```python
from build123d import *

# Parameters (mm, degrees)
SKETCH2_R                       = 80
SKETCH2_R_2                     = 31
BOSS_EXTRUDE1_DEPTH             = 5
F_4_0MM_DOWEL_HOLE1_D           = 4
F_4_0MM_DOWEL_HOLE1_CSINK_D     = 4.05
F_4_0MM_DOWEL_HOLE1_CSINK_ANGLE = 90
F_3_0MM_DOWEL_HOLE1_D           = 3
F_3_0MM_DOWEL_HOLE1_CSINK_D     = 3.05
F_3_0MM_DOWEL_HOLE1_CSINK_ANGLE = 90
SKETCH13_R                      = 5
CUT_EXTRUDE1_DEPTH              = 3


with BuildPart() as part:
    # Sketch2 → Boss-Extrude1 (new body)
    with BuildSketch(Plane.XY):
        Circle(SKETCH2_R)
        Circle(SKETCH2_R_2, mode=Mode.SUBTRACT)
    extrude(amount=BOSS_EXTRUDE1_DEPTH)

    # Ø4.0mm Dowel Hole1 (through all)
    with Locations(Plane.XY.offset(5)):
        with Locations((0, 70), (-49.497474683, 49.497474683), (-70, 0), (-49.497474683, -49.497474683), (0, -70), (49.497474683, -49.497474683), (70, 0), (49.497474683, 49.497474683)):
            CounterSinkHole(F_4_0MM_DOWEL_HOLE1_D / 2, F_4_0MM_DOWEL_HOLE1_CSINK_D / 2, counter_sink_angle=F_4_0MM_DOWEL_HOLE1_CSINK_ANGLE)

    # Ø3.0mm Dowel Hole1 (through all)
    with Locations(Plane.XY.offset(5)):
        with Locations((0, 37), (-26.162950904, 26.162950904), (-37, 0), (-26.162950904, -26.162950904), (0, -37), (26.162950904, -26.162950904), (37, 0), (26.162950904, 26.162950904)):
            CounterSinkHole(F_3_0MM_DOWEL_HOLE1_D / 2, F_3_0MM_DOWEL_HOLE1_CSINK_D / 2, counter_sink_angle=F_3_0MM_DOWEL_HOLE1_CSINK_ANGLE)

    # Sketch13 → Cut-Extrude1 (cut)
    with BuildSketch(Plane.XY):
        with Locations((0, 37)):
            Circle(SKETCH13_R)
        with Locations((26.162950904, 26.162950904)):
            Circle(SKETCH13_R)
        with Locations((37, 0)):
            Circle(SKETCH13_R)
        with Locations((26.162950904, -26.162950904)):
            Circle(SKETCH13_R)
        with Locations((0, -37)):
            Circle(SKETCH13_R)
        with Locations((-26.162950904, -26.162950904)):
            Circle(SKETCH13_R)
        with Locations((-37, 0)):
            Circle(SKETCH13_R)
        with Locations((-26.162950904, 26.162950904)):
            Circle(SKETCH13_R)
    extrude(amount=CUT_EXTRUDE1_DEPTH, mode=Mode.SUBTRACT)


solid = part.part
```
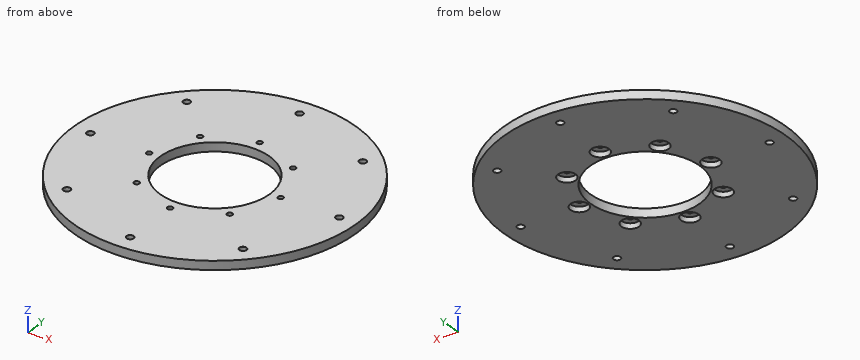
Input: part model. Units: mm. Frame: model coordinates. Give positions to 0.01 mm unless a question says otherwise; leave off trailing zeros. Order: outer loops, then holes, each group sorted by start corner. A loop starts at its lowest first (then second) coordinate and runs counter-clockwise, first axis right, second up. Notation, with made-up numbers: M 33.5,-17 L 91.5,-17 A19 cw 91.5,19 Z; hole C 72.5,45.5 d11. An arc over 180 degrees is marked long. Return JSON: item names as keys, results as strings.
1) Section query C-C on z = 0.9. Count the separate pieces of the cut face and the enclosed holes in it, and give its area (3 significant figures).
Taken from the geometry:
{"separate pieces": "1", "enclosed holes": "17", "area": "16,400 mm2"}
2) Section query D-D on x = -7. Output: boundary loops of the cut face in (y, z).
Taken from the geometry:
{"outline": "M -79.69,0 L -30.2,0 L -30.2,5 L -79.69,5 Z; M 30.2,0 L 79.69,0 L 79.69,5 L 30.2,5 Z"}
3) Section query A-A on y = 70. Output: boundary loops of the cut face in (x, z) (3 decimals), and give its area (3 significant figures).
Taken from the geometry:
{"outline": "M -38.73,0 L -2,0 L -2,4.975 L -2.025,5 L -38.73,5 Z; M 2,0 L 38.73,0 L 38.73,5 L 2.025,5 L 2,4.975 Z", "area": "367 mm2"}
4) Contact query for flat-ended pins moving along their axis: pin 1 (3 mm diameter, centred on x = 35, y = -1.5, fed in from -Z); pin 2 (2.5 mm diameter, centred on x = 0, y = 37, fed in from -Z); pin 3 (1 mm diameter, centred on y = 39.5, z = 4.5, fed in from -X); pin 4 (2 mm diameter, centred on y = 36.5, z = 0.5, fed in from +X). Output: stop coordinate, or through.
Taken from the geometry:
{"pin 1": "stops at z = 3", "pin 2": "passes through", "pin 3": "stops at x = -69.85", "pin 4": "stops at x = 71.69"}
5) Line query: L1, parallel to Y at x = 0, z = 3.6; L2, parallel to Y at x = 0, z = 0.75; L3, parallel to Y at x = 3.5, z = 2.7. Output: solid intervals per line, ascending. Write a range as [from, to].
Taken from the geometry:
{"L1": "y = [-80, -72], [-68, -38.5], [-35.5, -31], [31, 35.5], [38.5, 68], [72, 80]", "L2": "y = [-80, -72], [-68, -42], [-32, -31], [31, 32], [42, 68], [72, 80]", "L3": "y = [-79.92, -40.57], [-33.43, -30.8], [30.8, 33.43], [40.57, 79.92]"}
